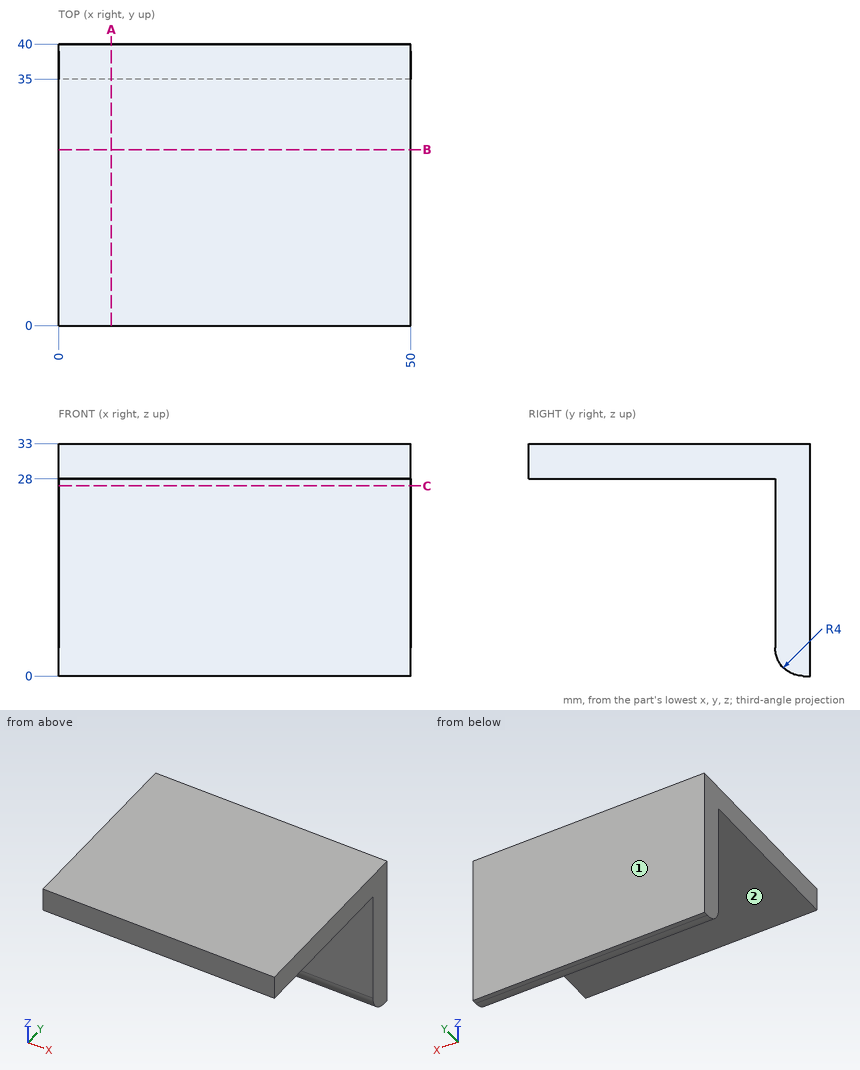
Source: three-view drawing plus pictorial views. Frame: mm from the lowest corner of the part. A direction names the side the tool comes from. Give positions to 0.01 mm unless a question says otherwise; leave off trailing zeros. Order: outer loops, then holes, each group sorted by start corner. A loop starts at its lowest first (then second) coordinate and runs counter-clockwise, first axis right, second up. Notation, with made-up numbers: (13, 43) -> (68, 43) arc R33 cw to (68, 72) -> close; hole circle Ø11 at (-34, 55.25). An arc over 180 degrees is marked (long way). Write each question's results on one line, items separated by ' | '. Start each with the question number.
Item 1: Cut plane A-A on x = 7.5. Return the cut outline in (y, z).
Item 2: Cut plane B-B on y = 25. Return the cut outline in (x, z), then the cut area to 3 significant figures.
Item 3: Line query: line 1 (Z direction, x = 40, y = 8); line 2 (Y direction, x = 33, z = 10); line 3 (Y direction, x = 46.5, z = 3). Output: solid intervals per line, ascending.
Item 4: Cut plane C-C on z = 27. Return the cut outline in (x, y).
Item 5: Set-up query: the marked faces 1 and 2. Return all of +Z, -Z, +X, -X, +Y, -Y with unobstructed straight access to the full face (end or side cutting, diameter ignored); none if empty.
Item 6: Contact query for flat-ended pins moving along their axis: P1, Ø3, axis at x = 22, z = 10.5, coming from the -Y side; P2, Ø5, axis at x = 36, y = 27, coming from the -Z side. Output: stop coordinate, or through.
Established:
1) outline: (0, 28) -> (35, 28) -> (35, 4) arc R4 ccw to (39, 0) -> (40, 0) -> (40, 33) -> (0, 33) -> close
2) outline: (0, 28) -> (50, 28) -> (50, 33) -> (0, 33) -> close | area: 250 mm^2
3) line 1: 28 to 33 | line 2: 35 to 40 | line 3: 35.13 to 40
4) outline: (0, 35) -> (50, 35) -> (50, 40) -> (0, 40) -> close
5) face 1: +Z, -Z, +X, -X, +Y | face 2: -Z, +X, -X, -Y
6) P1: y = 35 | P2: z = 28
